```python
from build123d import *

# Parameters (mm, degrees)
F3_ANGLE_BACK = 90
F3_ANGLE      = 180
F4_R          = 10
F5_DEPTH      = 50


with BuildPart() as f1:
    # F0 (on Top) → F1 (revolve)
    with BuildSketch(Plane.XY):
        with BuildLine():
            Line((-25, 0), (25, 0))
            ThreePointArc((25, 0), (0, 25), (-25, 0))
        make_face()
    revolve(axis=Axis((0, 0, 0), (1, 0, 0)))

    # F2 (on Front) → F3 (revolve)
    with BuildSketch(Plane.XZ, mode=Mode.PRIVATE) as f3_sk:
        with BuildLine():
            Line((-25, -50), (25, -50))
            ThreePointArc((25, -50), (0, -25), (-25, -50))
        make_face()
    revolve(f3_sk.sketch.rotate(Axis((0, 0, -50), (1, 0, 0)), -F3_ANGLE_BACK), axis=Axis((0, 0, -50), (1, 0, 0)), revolution_arc=F3_ANGLE)

    # F4 (on Top) → F5 (join)
    with BuildSketch(Plane.XY):
        Circle(F4_R)
    extrude(amount=-F5_DEPTH)


solid = f1.part
```
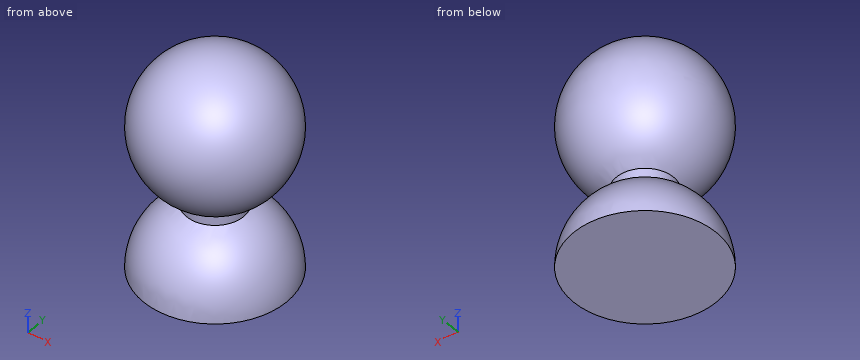
Could you check a few things on this model? Use its own coordinates, in mm. Coordinates: 2 decimals unless noted, no trailing zeros. Order: outer loops, then holes, each group sorted by start corner. A loop starts at its lowest first (then second) coordinate and runs counter-clockwise, first axis right, second up. Notation, with made-up numbers: M 56,-13 L 98,-13 A14 ccw 98,13 Z; hole C 39,12.25 d4. An arc over 180 degrees is marked long. Use one line per item in the form item = value. Start each with the question number.
1. For pin 1 (3 mm diameter, centred on y = -7, z = -34.5, fed in from -X); pin 2 (4 mm diameter, centred on y = -12, z = -8, fed in from +X); pin 3 (10 mm diameter, centred on x = 11, z = 11.5, fed in from +Y), each with a flat end and sliding along its axis, tell me the tip position at first contact or that it passes through.
2. Suppose I cut it at C-C on y = -15. Write out the boundary of the cut face in (x, z), then the cut area to 3 significant figures.
3. Suppose I cut it at A-A on y = 0. Write out the boundary of the cut face in (x, z), then the cut area to 3 significant figures.
4. Suppose I cut it at D-D on x = -19. Write out the boundary of the cut face in (y, z), then the cut area to 3 significant figures.
5. Please list where these lines run through material, in increasing order: line 1 (Z direction, x = 0, y = 14.5); line 2 (Z direction, x = 10.5, y = -6.5); line 3 (X direction, y = 17.5, z = -7.5).
Geometry says:
q1.pin_1 = -19.61
q1.pin_2 = 21.7
q1.pin_3 = 22.49
q2.outline = M -20,-50 L 20,-50 A20 ccw Z; C 0,0 d40
q2.area = 1,880 mm^2
q3.outline = M -25,-50 L 25,-50 A25 ccw 10,-27.09 L 10,-22.91 A25 ccw long -10,-22.91 L -10,-27.09 A25 ccw Z
q3.area = 2,970 mm^2
q4.outline = M -16.25,-50 L 16.25,-50 A16.25 ccw Z; C 0,0 d32.5
q4.area = 1,240 mm^2
q5.line_1 = -50 to -29.63, -20.37 to 20.37
q5.line_2 = -50 to -28.26, -21.74 to 21.74
q5.line_3 = -16.2 to 16.2
